Autodesk Fusion 360 part; units mm, degrees
sketch "Sketch1" plane through (0, 0, 0) normal (0, 0, 1) x (1, 0, 0)
  circle A0 centre (0, 0) radius 6.604
  line L0 (-12.827, 13.97) -> (36.703, 13.97)
  line L1 (36.703, 13.97) -> (36.703, -13.97)
  line L2 (36.703, -13.97) -> (-12.827, -13.97)
  line L3 (-12.827, -13.97) -> (-12.827, 13.97)
  line L4 (16.129, 10.287) -> (31.623, 10.287)
  line L5 (31.623, 10.287) -> (31.623, -10.287)
  line L6 (31.623, -10.287) -> (16.129, -10.287)
  line L7 (16.129, -10.287) -> (16.129, 10.287)
  line L8 (16.129, 0) -> (31.623, 0)
  point P0 (16.129, 0)
  point P1 (31.623, 0)
  point P2 (-12.827, 0)
  point P3 (36.703, 0)
  point P4 (23.876, 0)
  dimension "d1" = 13.208
  dimension "d2" = 15.494
  dimension "d3" = 20.574
  dimension "d4" = 23.876
  dimension "d5" = 5.08
  dimension "d6" = 49.53
  dimension "d7" = 27.94
extrude "Extrude1" add sketch "Sketch1" along normal blind 31.75
sketch "Sketch2" plane through (36.703, 0, 0) normal (1, 0, 0) x (0, 1, 0)
  line L0 (-13.97, 0) -> (13.97, 0)
  line L1 (13.97, 0) -> (13.97, 31.75)
  line L2 (13.97, 31.75) -> (-13.97, 31.75)
  line L3 (-13.97, 31.75) -> (-13.97, 0)
  line L4 (0, 0) -> (0, 40.147)
  circle A0 centre (0, 22.86) radius 2.286
  point P0 (0, 22.86)
  dimension "d10" = 8.89
  dimension "d11" = 4.572
extrude "Extrude2" cut sketch "Sketch2" against normal blind 7.62 contours L4 A0 | L4 A0
sketch "Sketch3" plane through (0, 0, 31.75) normal (0, 0, 1) x (-1, 0, 0)
  line L0 (-31.623, 10.287) -> (-16.129, 10.287)
  line L1 (-16.129, 10.287) -> (-16.129, -10.287)
  line L2 (-16.129, -10.287) -> (-31.623, -10.287)
  line L3 (-31.623, -10.287) -> (-31.623, 10.287)
  circle A0 centre (0, 0) radius 6.604
  line L4 (12.827, 13.97) -> (-36.703, 13.97)
  line L5 (-36.703, 13.97) -> (-36.703, -13.97)
  line L6 (-36.703, -13.97) -> (12.827, -13.97)
  line L7 (12.827, -13.97) -> (12.827, 13.97)
  line L8 (-7.493, -13.97) -> (-36.703, -13.97)
  line L9 (-36.703, -13.97) -> (-36.703, 13.97)
  line L10 (-36.703, 13.97) -> (-7.493, 13.97)
  line L11 (-7.493, 13.97) -> (-7.493, -13.97)
  dimension "d14" = 29.21
extrude "Extrude3" add sketch "Sketch3" along normal blind 82.55 contours L0 L1 L2 L3 | L4 L5 L6 L8 L9 L10 L11
sketch "Sketch4" plane through (0, 0, 114.3) normal (0, 0, 1) x (-1, 0, 0)
  line L0 (-7.493, 13.97) -> (-36.703, 13.97)
  line L1 (-36.703, 13.97) -> (-36.703, -13.97)
  line L2 (-36.703, -13.97) -> (-7.493, -13.97)
  line L3 (-7.493, -13.97) -> (-7.493, 13.97)
  line L4 (-36.703, -17.78) -> (-1.143, -17.78)
  line L5 (-1.143, -17.78) -> (-1.143, 17.78)
  line L6 (-1.143, 17.78) -> (-36.703, 17.78)
  line L7 (-36.703, 17.78) -> (-36.703, -17.78)
  line L8 (-36.703, -17.78) -> (-1.143, 17.78) construction
  line L9 (-1.143, -17.78) -> (-36.703, 17.78) construction
  line L10 (-36.703, -13.97) -> (-36.703, 13.97)
  point P0 (-18.923, 0)
  dimension "d17" = 35.56
  dimension "d18" = 35.56
extrude "Extrude4" add sketch "Sketch4" along normal blind 35.56
sketch "Sketch5" plane through (36.703, 0, 0) normal (1, 0, 0) x (0, 1, 0)
  circle A0 centre (0, 22.86) radius 2.286
  line L0 (-13.97, 0) -> (13.97, 0)
  line L1 (13.97, 0) -> (13.97, 114.3)
  line L2 (13.97, 114.3) -> (17.78, 114.3)
  line L3 (17.78, 114.3) -> (17.78, 149.86)
  line L4 (17.78, 149.86) -> (-17.78, 149.86)
  line L5 (-17.78, 149.86) -> (-17.78, 114.3)
  line L6 (-17.78, 114.3) -> (-13.97, 114.3)
  line L7 (-13.97, 114.3) -> (-13.97, 0)
  line L8 (-13.335, 145.415) -> (13.335, 145.415)
  line L9 (13.335, 145.415) -> (13.335, 118.745)
  line L10 (13.335, 118.745) -> (-13.335, 118.745)
  line L11 (-13.335, 118.745) -> (-13.335, 145.415)
  dimension "d21" = 4.445
  dimension "d22" = 4.445
  dimension "d23" = 4.445
  dimension "d24" = 4.445
extrude "Extrude5" cut sketch "Sketch5" against normal blind 45.72 contours L8 L9 L10 L11
The model under review builds one solid part; all positions refer to its coordinate system, in mm. A direction names the side the tool comes from. Round coordinates to 2 decimals unless told otherwise and drop trailing zeros. Order: outer loops, then holes, each group sorted by start corner. A loop starts at its lowest first (then second) coordinate and runs counter-clockwise, first axis right, second up. Notation, with made-up numbers: (-25.75, 50) -> (-4.75, 50) arc R20 cw to (-4.75, 57) -> close; hole circle Ø2 at (69, 13). An arc over 180 degrees is marked (long way). Use a Markdown table: item, result.
Q1. Mouldability with a two-part tool opening along X and no side actions: class faces 5 (the flat face through (-12.827, 0, 16)), 6 (the flat face through (24, -10.287, 16)), 7 (the flat face through (31.623, 0, 16)), 8 (the flat face through (19, 0, 145.415)) as +X half, -X half, draft (parallel to the pull), parting line (faces both ways), or undercut.
Values:
| item | result |
|---|---|
| face 5 | -X half |
| face 6 | undercut |
| face 7 | undercut |
| face 8 | draft |
Q2. We need section A-A on z = 128. Write out the cut boundary in (x, y) (3 decimals).
Values:
| item | result |
|---|---|
| outline | (1.143, -17.78) -> (36.703, -17.78) -> (36.703, -13.335) -> (1.143, -13.335) -> close; (1.143, 13.335) -> (36.703, 13.335) -> (36.703, 17.78) -> (1.143, 17.78) -> close |
Q3. We need section B-B on x = 4. Write out the cut boundary in (y, z) (3 decimals), then the cut area to 3 significant figures.
Values:
| item | result |
|---|---|
| outline | (-17.78, 114.3) -> (17.78, 114.3) -> (17.78, 149.86) -> (-17.78, 149.86) -> close; (-13.97, 0) -> (-5.255, 0) -> (-5.255, 31.75) -> (-13.97, 31.75) -> close; (5.255, 0) -> (13.97, 0) -> (13.97, 31.75) -> (5.255, 31.75) -> close; hole (-13.335, 118.745) -> (13.335, 118.745) -> (13.335, 145.415) -> (-13.335, 145.415) -> close |
| area | 1,110 mm^2 |
Q4. For line 1 (Z direction, x = 5.5, y = -8.5) (3 decimals); line 2 (Z direction, x = 35.35, y = 0) (3 decimals); line 3 (X direction, y = -8.5, z = 8.5), list the stretches that pass through material, from the lowest coordinate up.
Values:
| item | result |
|---|---|
| line 1 | z = 0 to 31.75, 114.3 to 118.745, 145.415 to 149.86 |
| line 2 | z = 0 to 20.574, 25.146 to 118.745, 145.415 to 149.86 |
| line 3 | x = -12.83 to 16.13, 31.62 to 36.7 |
Q5. Clearance check with flat-ended pins moving along their axes: P1, Ø5, axis at x = 16.5, z = 70, coming from the +Y side; P2, Ø7.5, axis at x = 24.5, z = 8, coming from the -Y side. State where each tip first meets the part, or that it passes through.
Values:
| item | result |
|---|---|
| P1 | stops at y = 13.97 |
| P2 | stops at y = -13.97 |
Q6. We need section D-D on y = 0. Write out the cut boundary in (x, z) (3 decimals).
Values:
| item | result |
|---|---|
| outline | (-12.827, 0) -> (-6.604, 0) -> (-6.604, 31.75) -> (-12.827, 31.75) -> close; (1.143, 114.3) -> (7.493, 114.3) -> (7.493, 31.75) -> (6.604, 31.75) -> (6.604, 0) -> (16.129, 0) -> (16.129, 31.75) -> (31.623, 31.75) -> (31.623, 25.146) -> (36.703, 25.146) -> (36.703, 118.745) -> (1.143, 118.745) -> close; (1.143, 145.415) -> (36.703, 145.415) -> (36.703, 149.86) -> (1.143, 149.86) -> close; (31.623, 0) -> (36.703, 0) -> (36.703, 20.574) -> (31.623, 20.574) -> close |
Q7. Tool access review of faces 1 (the flat face through (24, 0, 31.75)), 2 (the flat face through (-7, 0, 31.75)), 3 (the flat face through (17, 13.97, 44)), 4 (the flat face through (1.143, -16, 132)): name each direction out of +Z, -Z, +X, -X, +Y, -Y from which nothing blocks a thin tool from reaching the whole face with its end or side.
Values:
| item | result |
|---|---|
| face 1 | -Z |
| face 2 | -X, +Y, -Y |
| face 3 | -Z, +X, -X, +Y |
| face 4 | +Z, -X, +Y, -Y |
Q8. We need section C-C on z = 22.86. Write out the cut boundary in (x, y), then the cut area to 3 significant figures.
Values:
| item | result |
|---|---|
| outline | (-12.83, -13.97) -> (36.7, -13.97) -> (36.7, -2.29) -> (31.62, -2.29) -> (31.62, -10.29) -> (16.13, -10.29) -> (16.13, 10.29) -> (31.62, 10.29) -> (31.62, 2.29) -> (36.7, 2.29) -> (36.7, 13.97) -> (-12.83, 13.97) -> close; hole circle Ø13.21 at (0, 0) |
| area | 905 mm^2 |
